```python
from build123d import *

# Parameters (mm, degrees)
SKETCH3_W           = 18
SKETCH3_H           = 6
BOSS_EXTRUDE1_DEPTH = 2
SKETCH4_R           = 1.75
CUT_EXTRUDE1_DEPTH  = 3
SKETCH5_W           = 18
SKETCH5_H           = 4.86
BOSS_EXTRUDE4_DEPTH = 2
SKETCH6_W           = 2
SKETCH6_H           = 10.86
BOSS_EXTRUDE5_DEPTH = 11.6
SKETCH7_W           = 10.86
SKETCH7_H           = 3.7
BOSS_EXTRUDE6_DEPTH = 5.5
CUT_EXTRUDE2_DEPTH  = 4.7


with BuildPart() as part:
    # Sketch3 → Boss-Extrude1 (new body)
    with BuildSketch(Plane(origin=(0, 0, 0), x_dir=(1, 0, 0), z_dir=(0, 1, 0))):
        Rectangle(SKETCH3_W, SKETCH3_H)
    extrude(amount=BOSS_EXTRUDE1_DEPTH)

    # Sketch4 → Cut-Extrude1 (cut, through all)
    with BuildSketch(Plane(origin=(0, 2, 0), x_dir=(1, 0, 0), z_dir=(0, 1, 0))):
        with Locations((-5.01, 0)):
            Circle(SKETCH4_R)
        with Locations((5.01, 0)):
            Circle(SKETCH4_R)
    extrude(amount=-CUT_EXTRUDE1_DEPTH, mode=Mode.SUBTRACT)

    # Sketch5 → Boss-Extrude4 (add)
    with BuildSketch(Plane(origin=(0, 0, 0), x_dir=(1, 0, 0), z_dir=(0, 1, 0))):
        with Locations((0, -5.43)):
            Rectangle(SKETCH5_W, SKETCH5_H)
    boss_extrude4 = extrude(amount=BOSS_EXTRUDE4_DEPTH)

    # Sketch6 → Boss-Extrude5 (add)
    with BuildSketch(Plane.XZ):
        with Locations((-8, 2.43)):
            Rectangle(SKETCH6_W, SKETCH6_H)
    boss_extrude5 = extrude(amount=BOSS_EXTRUDE5_DEPTH)

    # Sketch7 → Boss-Extrude6 (add)
    with BuildSketch(Plane.ZY.offset(9)):
        with Locations((2.43, -9.75)):
            Rectangle(SKETCH7_W, SKETCH7_H)
    boss_extrude6 = extrude(amount=BOSS_EXTRUDE6_DEPTH)

    # Sketch8 → Cut-Extrude2 (cut, through all)
    with BuildSketch(Plane(origin=(0, -7.9, 0), x_dir=(1, 0, 0), z_dir=(0, 1, 0))):
        with BuildLine():
            Line((-11.05, -0.43), (-11.05, -4.43))
            ThreePointArc((-11.05, -4.43), (-12, -5.38), (-12.95, -4.43))
            Line((-12.95, -4.43), (-12.95, -0.43))
            ThreePointArc((-12.95, -0.43), (-12, 0.52), (-11.05, -0.43))
        make_face()
    cut_extrude2 = extrude(amount=-CUT_EXTRUDE2_DEPTH, mode=Mode.SUBTRACT)

    # Mirror1: Boss-Extrude4, Boss-Extrude5, Boss-Extrude6, Cut-Extrude2 across plane
    add(boss_extrude4.mirror(Plane(origin=(0, 0, 0), x_dir=(0, 0, 1), z_dir=(1, 0, 0))))
    add(boss_extrude5.mirror(Plane(origin=(0, 0, 0), x_dir=(0, 0, 1), z_dir=(1, 0, 0))))
    add(boss_extrude6.mirror(Plane(origin=(0, 0, 0), x_dir=(0, 0, 1), z_dir=(1, 0, 0))))
    add(cut_extrude2.mirror(Plane(origin=(0, 0, 0), x_dir=(0, 0, 1), z_dir=(1, 0, 0))), mode=Mode.SUBTRACT)


solid = part.part
```
Geometry check sheet. Reference: the model listing, model coordinates, mm. A direction names the side the tool comes from. Round coordinates to 2 decimals unless told otherwise and drop trailing zeros. Order: outer loops, then holes, each group sorted by start corner. A loop starts at its lowest first (then second) coordinate and runs counter-clockwise, first axis right, second up. Notation, with made-up numbers: M -32,-12.75 L 10,-12.75 A7 ccw 10,-1.75 Z; hole C 89,-21.5 d11. An arc over 180 degrees is marked long. Write item = value, one per line.
Q1. Release check for a two-part mould opening along X. For faces 6 (the flat face through (-9, -3, 2)), 7 (the cylindrical face through (-12.02, -9.72, -0.52)), 8 (the flat face through (0, 2, 2)) record: released by +X, released by -X, zero draft, split by the parting line, or undercut.
Answer block:
face_6 = released by -X
face_7 = undercut
face_8 = zero draft
Q2. Section check A-A (y = -4.75). Enter the section's corners in (x, z), plus the area to 3 significant figures.
Answer block:
outline = M -9,-3 L -7,-3 L -7,7.86 L -9,7.86 Z; M 7,-3 L 9,-3 L 9,7.86 L 7,7.86 Z
area = 43.4 mm^2
Q3. Depth check by flat-ended pin: pin 1 Ø1.6 at (x, z) = (-11, 0) entering from +Y; pin 2 Ø6 at (x, z) = (1, 0) entering from -Y; pin 3 Ø3 at (y, z) = (-1, 0.5) entering from -X. Enter the tip coordinate at first touch or a pass-through.
Answer block:
pin_1 = -7.9
pin_2 = 0
pin_3 = -9
Q4. Section check C-C (z = 2.25). Enter the section's corners in (x, y).
Answer block:
outline = M -14.5,-11.6 L -12.95,-11.6 L -12.95,-7.9 L -14.5,-7.9 Z; M -11.05,-11.6 L -7,-11.6 L -7,0 L 7,0 L 7,-11.6 L 11.05,-11.6 L 11.05,-7.9 L 9,-7.9 L 9,2 L -9,2 L -9,-7.9 L -11.05,-7.9 Z; M 12.95,-11.6 L 14.5,-11.6 L 14.5,-7.9 L 12.95,-7.9 Z
Q5. Scan lines: line 1 (X direction, y = 1.4, z = 0); line 2 (X direction, y = -8.5, z = 4); line 3 (Z direction, x = 5.01, y = 0.5). Record each from-to range of solid material in increasing order.
Answer block:
line_1 = -9 to -6.76, -3.26 to 3.26, 6.76 to 9
line_2 = -14.5 to -12.95, -11.05 to -7, 7 to 11.05, 12.95 to 14.5
line_3 = -3 to -1.75, 1.75 to 7.86
Q6. Set-up check for faces 1 (the flat face through (7, -6, 2)), 2 (the flat face through (9, -3, 2)), 3 (the flat face through (1, 0.2, -3)), 4 (the flat face through (-10, -7.9, 2)), 5 (the flat face through (11.05, -10, 2)): record each of +Z, -Z, +X, -X, +Y, -Y from which the full face is reachable in a straight line by a thin tool's end or side.
Answer block:
face_1 = +Z, -Z, -Y
face_2 = +Z, -Z, +X, +Y
face_3 = -Z, +X, -X, +Y, -Y
face_4 = +Z, -Z, -X, +Y
face_5 = +Y, -Y
Q7. Section check B-B (x = -12). Enter the section's corners in (y, z).
Answer block:
outline = M -11.6,-3 L -7.9,-3 L -7.9,-0.52 L -11.6,-0.52 Z; M -11.6,5.38 L -7.9,5.38 L -7.9,7.86 L -11.6,7.86 Z
Q8. Section check D-D (z = 0). Enter the section's corners in (x, y).
Answer block:
outline = M -14.5,-11.6 L -12.85,-11.6 L -12.85,-7.9 L -14.5,-7.9 Z; M -11.15,-11.6 L -7,-11.6 L -7,0 L -6.76,0 L -6.76,2 L -9,2 L -9,-7.9 L -11.15,-7.9 Z; M -3.26,0 L 3.26,0 L 3.26,2 L -3.26,2 Z; M 6.76,0 L 7,0 L 7,-11.6 L 11.15,-11.6 L 11.15,-7.9 L 9,-7.9 L 9,2 L 6.76,2 Z; M 12.85,-11.6 L 14.5,-11.6 L 14.5,-7.9 L 12.85,-7.9 Z
